CAD build for the part. Positions are in the model's coordinates, mm. A direction names the side the tool comes from. Coordinates: 2 decimals unless noted, no trailing zeros. Loops run counter-clockwise (first coordinate to the right, second up) from the corner with the lowest first, then second, coordinate; pieces in that order, holes last. Notation, with made-up numbers: (17.25, 58) -> (25.25, 58) arc R24 cw to (25.25, 72) -> close; hole circle Ø3 at (52.25, 59). An arc over 180 degrees is marked (long way). Answer as CSV lines item,"result". Start each with the question number.
from build123d import *

# Parameters (mm, degrees)
SKETCH_1_W                  = 15
SKETCH_1_H                  = 15
SKETCH_1_W_2                = 12
SKETCH_1_H_2                = 12
EXTRUDE_1_DEPTH             = 600
SKETCH_3_R                  = 2.25
CUT_EXTRUDE_2_DEPTH         = 25
SKETCH_4_R                  = 2.7
CUT_EXTRUDE_3_DEPTH         = 20
SKETCH_6_R                  = 2.1
CUT_EXTRUDE_4_DEPTH         = 20
SKETCH_9_R                  = 5
CUT_EXTRUDE_7_DEPTH         = 10
SKETCH_10_R                 = 2.7
CUT_EXTRUDE_8_DEPTH         = 30
SKETCH_11_R                 = 5
CUT_EXTRUDE_9_DEPTH         = 10
HOLE_WIZARD_10_0_10_1_D     = 10
HOLE_WIZARD_10_0_10_1_DEPTH = 1.5


with BuildPart() as part:
    # ｽｹｯﾁ1 → ﾎﾞｽ - 押し出し1 (new body)
    with BuildSketch(Plane.XY):
        Rectangle(SKETCH_1_W, SKETCH_1_H)
        Rectangle(SKETCH_1_W_2, SKETCH_1_H_2, mode=Mode.SUBTRACT)
    extrude(amount=EXTRUDE_1_DEPTH)

    # ｽｹｯﾁ3 → ｶｯﾄ - 押し出し2 (cut)
    with BuildSketch(Plane(origin=(0, 7.5, 0), x_dir=(1, 0, 0), z_dir=(0, 1, 0))):
        with Locations((0, -7.5)):
            Circle(SKETCH_3_R)
        with Locations((0, -592.5)):
            Circle(SKETCH_3_R)
    extrude(amount=-CUT_EXTRUDE_2_DEPTH, mode=Mode.SUBTRACT)

    # ｽｹｯﾁ4 → ｶｯﾄ - 押し出し3 (cut)
    with BuildSketch(Plane(origin=(7.5, 0, 0), x_dir=(0, 0, -1), z_dir=(1, 0, 0))):
        with Locations((-536, 0)):
            Circle(SKETCH_4_R)
        with Locations((-501, 0)):
            Circle(SKETCH_4_R)
        with Locations((-99, 0)):
            Circle(SKETCH_4_R)
        with Locations((-64, 0)):
            Circle(SKETCH_4_R)
    extrude(amount=-CUT_EXTRUDE_3_DEPTH, mode=Mode.SUBTRACT)

    # ｽｹｯﾁ6 → ｶｯﾄ - 押し出し4 (cut)
    with BuildSketch(Plane(origin=(0, 7.5, 0), x_dir=(1, 0, 0), z_dir=(0, 1, 0))):
        with Locations((0, -336.5)):
            Circle(SKETCH_6_R)
        with Locations((0, -263.5)):
            Circle(SKETCH_6_R)
    extrude(amount=-CUT_EXTRUDE_4_DEPTH, mode=Mode.SUBTRACT)

    # ｽｹｯﾁ9 → ｶｯﾄ - 押し出し7 (cut)
    with BuildSketch(Plane.XZ.offset(7.5)):
        with Locations((0, 592.5)):
            Circle(SKETCH_9_R)
        with Locations((0, 336.5)):
            Circle(SKETCH_9_R)
        with Locations((0, 263.5)):
            Circle(SKETCH_9_R)
        with Locations((0, 7.5)):
            Circle(SKETCH_9_R)
    extrude(amount=-CUT_EXTRUDE_7_DEPTH, mode=Mode.SUBTRACT)

    # ｽｹｯﾁ10 → ｶｯﾄ - 押し出し8 (cut)
    with BuildSketch(Plane(origin=(0, -7.5, 0), x_dir=(-1, 0, 0), z_dir=(0, -1, 0))):
        with Locations((0, -40)):
            Circle(SKETCH_10_R)
        with Locations((0, -77)):
            Circle(SKETCH_10_R)
        with Locations((0, -523)):
            Circle(SKETCH_10_R)
        with Locations((0, -560)):
            Circle(SKETCH_10_R)
    extrude(amount=-CUT_EXTRUDE_8_DEPTH, mode=Mode.SUBTRACT)

    # ｽｹｯﾁ11 → ｶｯﾄ - 押し出し9 (cut)
    with BuildSketch(Plane(origin=(0, 7.5, 0), x_dir=(1, 0, 0), z_dir=(0, 1, 0))):
        with Locations((0, -40)):
            Circle(SKETCH_11_R)
        with Locations((0, -77)):
            Circle(SKETCH_11_R)
        with Locations((0, -560)):
            Circle(SKETCH_11_R)
        with Locations((0, -523)):
            Circle(SKETCH_11_R)
    extrude(amount=-CUT_EXTRUDE_9_DEPTH, mode=Mode.SUBTRACT)

    # Ø10.0 (10) 直径の穴1
    with Locations(Plane.ZY.offset(7.5)):
        with Locations((64, 0), (99, 0), (501, 0), (536, 0)):
            Hole(HOLE_WIZARD_10_0_10_1_D / 2, depth=HOLE_WIZARD_10_0_10_1_DEPTH)


solid = part.part
Item 1: Saw through at B-B (y = 0). Count the separate pieces of the cut face and the enclosed holes in it, plus the area to 3 significant figures.
Item 2: Saw through at A-A (z = 137.5). Write the cut outline in (x, y), plus the area to 3 significant figures.
Item 3: Two-plate mould, pull along Z, no slides. Class faces 5 (the face through (-7, 0, 0)), 6 (the face through (-0.651, -6.76, 597.457)), 7 (the face through (-7.5, 0, 296)): pulls with the +Z half, pulls with the -Z half, needs draft (parallel to the pull), parting line crosses it, or undercut.
Item 4: Wall check: probe 1 along X at (y, z) = (-3.75, 365); probe 2 along X at (y, z) = (-6.9, 40). Give the ranges that are in metal, low to high.
Item 5: Which spindle directions (+Z, -Z, +X, -X, +Y, -Y) get a long thin tool onto all of the face, cutting with end or side? Do faces 1 (the face through (-6.74, -1.915, 94.381)), 2 (the face through (-0.651, -6.76, 268.457)), 3 (the face through (-6, 0, 296)), 4 (the face through (-1.08, 6.76, 81.88)). Say none if no direction does.
Item 6: Flat gauge pins, fed straight in: pin 1 Ø5 at (x, y) = (1.5, 1) entering from -Z; pin 2 Ø8 at (x, z) = (0, 560) entering from +Y; pin 3 Ø1.5 at (x, y) = (5.5, -3.5) entering from +Z; pin 4 Ø8 at (x, z) = (0, 263.5) entering from -Y. Where does each tip first touch, or does it go through?
Geometry check:
1,separate pieces,"10"
1,enclosed holes,"0"
1,area,"1,710 mm2"
2,outline,"(-7.5, -7.5) -> (7.5, -7.5) -> (7.5, 7.5) -> (-7.5, 7.5) -> close; hole (-6, -6) -> (6, -6) -> (6, 6) -> (-6, 6) -> close"
2,area,"81.0 mm2"
3,face 5,"pulls with the -Z half"
3,face 6,"undercut"
3,face 7,"needs draft"
4,probe 1,"-7.5 to -6, 6 to 7.5"
4,probe 2,"-7.5 to -2.7, 2.7 to 7.5"
5,face 1,"-X"
5,face 2,"-Y"
5,face 3,"+Z, -Z"
5,face 4,"+Y"
6,pin 1,"through"
6,pin 2,"y = -6"
6,pin 3,"z = 600"
6,pin 4,"y = 6"
